```python
from build123d import *

# Parameters (mm, degrees)
CROQUIS1_R                 = 50
SALIENTE_EXTRUIR1_DEPTH    = 5
CROQUIS2_R                 = 1.5
CORTAR_EXTRUIR1_DEPTH      = 5
CROQUIS3_R                 = 3.5
CORTAR_EXTRUIR2_DEPTH      = 3
MATRIZC2_COUNT             = 3
CROQUIS4_R                 = 3
SALIENTE_EXTRUIR2_DEPTH    = 5
CROQUIS6_R                 = 2.55
SALIENTE_EXTRUIR4_DEPTH    = 2
SALIENTE_EXTRUIR5_DEPTH    = 12
CORTAR_EXTRUIR3_DEPTH      = 99.269119567
CORTAR_EXTRUIR3_DEPTH_BACK = 25
CROQUIS8_W                 = 8
CROQUIS8_H                 = 5
CROQUIS9_W                 = 5
CROQUIS9_H                 = 1.5
CORTAR_EXTRUIR4_DEPTH      = 11
REDONDEO1_R                = 1.5
CROQUIS10_R                = 3
SALIENTE_EXTRUIR6_DEPTH    = 5
CROQUIS5_R                 = 1.25
SALIENTE_EXTRUIR7_DEPTH    = 5
CROQUIS12_R                = 1.05
SALIENTE_EXTRUIR8_DEPTH    = 5
CROQUIS11_R                = 2.5
SALIENTE_EXTRUIR9_DEPTH    = 4
CROQUIS13_R                = 1
SALIENTE_EXTRUIR10_DEPTH   = 5


with BuildPart() as part:
    # Croquis1 → Saliente-Extruir1 (new body)
    with BuildSketch(Plane(origin=(0, 0, 0), x_dir=(1, 0, 0), z_dir=(0, 1, 0))):
        with Locations(Location((0, 0, 0), (0, 0, 270))):
            Circle(CROQUIS1_R)
    extrude(amount=SALIENTE_EXTRUIR1_DEPTH)

    # Croquis2 → Cortar-Extruir1 (cut)
    with BuildSketch(Plane(origin=(0, 5, 0), x_dir=(1, 0, 0), z_dir=(0, 1, 0))):
        with Locations(Location((44.5, 0, 0), (0, 0, 270))):
            Circle(CROQUIS2_R)
    cortar_extruir1 = extrude(amount=-CORTAR_EXTRUIR1_DEPTH, mode=Mode.SUBTRACT)

    # Croquis3 → Cortar-Extruir2 (cut)
    with BuildSketch(Plane(origin=(0, 5, 0), x_dir=(1, 0, 0), z_dir=(0, 1, 0))):
        with Locations(Location((44.5, 0, 0), (0, 0, 270))):
            Circle(CROQUIS3_R)
    cortar_extruir2 = extrude(amount=-CORTAR_EXTRUIR2_DEPTH, mode=Mode.SUBTRACT)

    # MatrizC2: Cortar-Extruir1, Cortar-Extruir2 ×3 about axis
    matrizc2_axis = Axis((0, 0, 0), (0, 1, 0))
    add([cortar_extruir1.rotate(matrizc2_axis, i * 360 / MATRIZC2_COUNT) for i in range(1, MATRIZC2_COUNT)], mode=Mode.SUBTRACT)
    add([cortar_extruir2.rotate(matrizc2_axis, i * 360 / MATRIZC2_COUNT) for i in range(1, MATRIZC2_COUNT)], mode=Mode.SUBTRACT)

    # Croquis4 → Saliente-Extruir2 (add)
    with BuildSketch(Plane.XZ):
        with Locations(Location((-32, 14.7, 0), (0, 0, 90))):
            Circle(CROQUIS4_R)
        with Locations(Location((-32, -14.7, 0), (0, 0, 90))):
            Circle(CROQUIS4_R)
    extrude(amount=SALIENTE_EXTRUIR2_DEPTH)

    # Croquis6 → Saliente-Extruir4 (add)
    with BuildSketch(Plane.XZ):
        with Locations(Location((27.173827718, 5.816127145, 0), (0, 0, 90))):
            Circle(CROQUIS6_R)
        with Locations(Location((37.323827718, -11.764188552, 0), (0, 0, 90))):
            Circle(CROQUIS6_R)
        with Locations(Location((-14.51663522, -18.253872855, 0), (0, 0, 90))):
            Circle(CROQUIS6_R)
        with Locations(Location((-4.36663522, -35.834188552, 0), (0, 0, 90))):
            Circle(CROQUIS6_R)
    extrude(amount=SALIENTE_EXTRUIR4_DEPTH)

    # Croquis7 → Saliente-Extruir5 (add)
    with BuildSketch(Plane.XZ):
        Polygon((2.190063509, 1.20669873), (23.840698604, 13.70669873), (18.340698604, 23.232978171), (-3.309936491, 10.732978171), align=None)
    extrude(amount=SALIENTE_EXTRUIR5_DEPTH)

    # Croquis8 → Cortar-Extruir3 (cut, two sides: drawn at the far end of the back side and taken through both)
    with BuildSketch(Plane(origin=(23.815698604, 0, 13.75), x_dir=(0.49999999999999806, 0, -0.8660254037844398), z_dir=(0.8660254037844397, 0, 0.499999999999998)).offset(-CORTAR_EXTRUIR3_DEPTH_BACK)):
        with Locations((-5.45, -9.5)):
            Rectangle(CROQUIS8_W, CROQUIS8_H)
    extrude(amount=CORTAR_EXTRUIR3_DEPTH + CORTAR_EXTRUIR3_DEPTH_BACK, mode=Mode.SUBTRACT)

    # Croquis9 → Cortar-Extruir4 (cut)
    with BuildSketch(Plane(origin=(-5.475, 0, 9.482978171), x_dir=(0.8660254037844398, 0, 0.49999999999999806), z_dir=(-0.499999999999998, 0, 0.8660254037844397))):
        with Locations((7.5, -4)):
            Rectangle(CROQUIS9_W, CROQUIS9_H)
        with Locations((22.5, -4)):
            Rectangle(CROQUIS9_W, CROQUIS9_H)
    extrude(amount=-CORTAR_EXTRUIR4_DEPTH, mode=Mode.SUBTRACT)

    # Redondeo1
    redondeo1_edges = [part.edges().sort_by_distance(p)[0] for p in [
        (8.265381057, -7, 15.683940066),
        (12.265381057, -7, 8.755736835),
    ]]
    fillet(redondeo1_edges, radius=REDONDEO1_R)

    # Croquis10 → Saliente-Extruir6 (add)
    with BuildSketch(Plane.XZ):
        with Locations(Location((9.016660498, 36.382685902, 0), (0, 0, 90))):
            Circle(CROQUIS10_R)
        with Locations(Location((-25.624355653, 16.382685902, 0), (0, 0, 90))):
            Circle(CROQUIS10_R)
    extrude(amount=SALIENTE_EXTRUIR6_DEPTH)

    # Croquis5 → Saliente-Extruir7 (add)
    with BuildSketch(Plane.XZ.offset(5)):
        with Locations(Location((9.016660498, 36.382685902, 0), (0, 0, 270))):
            Circle(CROQUIS5_R)
        with Locations(Location((-25.624355653, 16.382685902, 0), (0, 0, 270))):
            Circle(CROQUIS5_R)
        with Locations(Location((-32, 14.7, 0), (0, 0, 270))):
            Circle(CROQUIS5_R)
        with Locations(Location((-32, -14.7, 0), (0, 0, 270))):
            Circle(CROQUIS5_R)
    extrude(amount=SALIENTE_EXTRUIR7_DEPTH)

    # Croquis12 → Saliente-Extruir8 (add)
    with BuildSketch(Plane.XZ.offset(2)):
        with Locations(Location((27.173827718, 5.816127145, 0), (0, 0, 270))):
            Circle(CROQUIS12_R)
        with Locations(Location((37.323827718, -11.764188552, 0), (0, 0, 270))):
            Circle(CROQUIS12_R)
        with Locations(Location((-4.36663522, -35.834188552, 0), (0, 0, 270))):
            Circle(CROQUIS12_R)
        with Locations(Location((-14.51663522, -18.253872855, 0), (0, 0, 270))):
            Circle(CROQUIS12_R)
    extrude(amount=SALIENTE_EXTRUIR8_DEPTH)

    # Croquis11 → Saliente-Extruir9 (add)
    with BuildSketch(Plane.XZ):
        with Locations(Location((15.322510954, -35.239367471, 0), (0, 0, 90))):
            Circle(CROQUIS11_R)
        with Locations(Location((22.856931966, -30.889367471, 0), (0, 0, 90))):
            Circle(CROQUIS11_R)
    extrude(amount=SALIENTE_EXTRUIR9_DEPTH)

    # Croquis13 → Saliente-Extruir10 (add)
    with BuildSketch(Plane.XZ.offset(4)):
        with Locations(Location((22.856931966, -30.889367471, 0), (0, 0, 270))):
            Circle(CROQUIS13_R)
        with Locations(Location((15.322510954, -35.239367471, 0), (0, 0, 270))):
            Circle(CROQUIS13_R)
    extrude(amount=SALIENTE_EXTRUIR10_DEPTH)


solid = part.part
```
For this review, take the finished solid that the model builds, in its own axes (mm). A direction names the side the tool comes from. Give positions to 0.01 mm unless a question says otherwise; leave off trailing zeros. Write each loop counter-clockwise with the first axis right and the second up, starting at its lowest first coordinate (ties: lowest second). Pieces come first, ordered by that corner, then holes. Notation, with made-up numbers: M 68.5,17 L 126.5,17 A30 ccw 126.5,49 Z; hole C -33.75,79 d4. An arc over 180 degrees is marked long. One line per item, written item: value.
1) The part is to be moulded in two halves that separate along Y. For faces 1 (the cylindrical face through (-21.2, 3.5, -35.2)), 2 (the flat face through (17, -3.25, 16)), 3 (the flat face through (4, -3.25, 9)), 4 (the flat face through (13, -12, 8)), say which applies: +Y half, -Y half, draft (parallel to the pull), parting line (faces both ways), or undercut.
Results are:
face 1: draft
face 2: undercut
face 3: undercut
face 4: -Y half
2) For P1, Ø8, axis at y = -2.5, z = -30, coming from the -X side; P2, Ø2.5, axis at x = 14.5, z = -36, coming from the -Y side; P3, Ø6.5, axis at x = -32.5, z = 15.5, coming from the -Y side; P4, Ø2.5, axis at x = 44.5, z = 0, coming from the +Y side, all flat-tipped, find the tip position at first contact; note any pin that passes through.
Results are:
P1: stops at x = -42.16
P2: stops at y = -9
P3: stops at y = -10
P4: passes through
3) Take a section at C-C, the plane x = -42.5. Write out the cut boundary in (y, z), then the cut area to 3 significant figures.
Results are:
outline: M 0,-26.34 L 5,-26.34 L 5,26.34 L 0,26.34 Z
area: 263 mm²
4) Take a section at B-B, the plane x = -32. Write out the cut boundary in (y, z).
Results are:
outline: M -10,-15.95 L -5,-15.95 L -5,-17.7 L 0,-17.7 L 0,-38.42 L 5,-38.42 L 5,38.42 L 0,38.42 L 0,17.7 L -5,17.7 L -5,15.95 L -10,15.95 L -10,13.45 L -5,13.45 L -5,11.7 L 0,11.7 L 0,-11.7 L -5,-11.7 L -5,-13.45 L -10,-13.45 Z
5) For line 1 (X direction, y = 1.6, z = 0); line 2 (X direction, y = 4.15, z = 0); line 3 (Y direction, x = 9.5, z = -10), list the stretches that pass through material, from the lowest coordinate up. Write a range as from..to.
Results are:
line 1: x = -50..43, 46..50
line 2: x = -50..41, 48..50
line 3: y = 0..5
6) Take a section at A-A, the plane z = 0. Write out the cut boundary in (x, y), then the cut area to 3 significant figures.
Results are:
outline: M -50,0 L 43,0 L 43,2 L 41,2 L 41,5 L -50,5 Z; M 46,0 L 50,0 L 50,5 L 48,5 L 48,2 L 46,2 Z
area: 473 mm²
7) For faces 5 (the cylindrical face through (48, 4, 0)), 6 (the flat face through (23.4, -4, -29.8)), 7 (the flat face through (9, -10, 36)), 8 (the cylindrical face through (43, 1, 0)), list the 3-axis set-ups (+Z, -Z, +X, -X, +Y, -Y) from which the entire face can be reached by the end or side of a thin tool; tool diameter is ignored.
Results are:
face 5: +Y
face 6: -Y
face 7: +Z, +X, -X, -Y
face 8: +Y, -Y
